Input: part model. Units: mm. Frame: model coordinates. A direction names the side the tool comes from. Round coordinates to 2 decimals unless told otherwise and drop trailing zeros. Loops run counter-clockwise (first coordinate to the right, second up) from the corner with the lowest first, then second, coordinate; pieces in that order, holes last.
1) Ray query, line 1 along Y through (x, z) = (0, 19); line 2 along X through (y, z) = (12.7, 40); line 3 along Y through (x, z) = (-2.5, 31). Return the intervals inside material, ascending.
2) Section B-B, the plane x = 3. Return loops of the section in (y, z), and give its area (3 significant figures).
3) Section D-D, the plane y = 17. Return loops of the section in (x, z), and give its area (3 significant figures).
4) Section A-A, the plane z = 41.5. Return loops of the section in (x, y).
5) Section C-C, the plane y = 21.5. Return loops of the section in (x, z).
6) Draft query along Y for faces 6 (the face through (0, 9.19, 36)), 7 (the face through (0, 27, 30)), 8 (the face through (0, 20.85, 36)). Return one class per face: pulls with the +Y half, pulls with the -Y half, needs draft (parallel to the pull), parting line crosses it, or undercut.
7) First-contact query: pin 1 (3 mm diameter, centred on y = 24.5, z = 33, fed in from -X); pin 2 (2 mm diameter, centred on x = 7, z = 7, fed in from -Y); pin 3 (3 mm diameter, centred on x = 4.5, y = 24.5, fed in from +Z); pin 4 (6 mm diameter, centred on x = 3, y = 19, fed in from -Z). Flat tips, straight axial feed; report the tip coordinate or a pass-through.
8) Access query for faces 1 (the face through (0, 14.85, 36)), 2 (the face through (0.657, 22.857, 12.325)), 3 (the face through (0, 9, 30)), 4 (the face through (-5, 24, 35)), 5 (the face through (0, 18, 30)). Directions: +Z, -Z, +X, -X, +Y, -Y. A direction counts if a zero-diameter tool reaches every point of the face in a straight line with its end or side. Return the directions, or none.
from build123d import *

# Parameters (mm, degrees)
SKETCH_1_R          = 10
EXTRUDE_1_DEPTH     = 30
SKETCH_2_W          = 10
SKETCH_2_H          = 17.320508075
EXTRUDE_3_DEPTH     = 15
CUT_EXTRUDE_1_DEPTH = 50.731328966
CUT_EXTRUDE_2_DEPTH = 50.731328966
CUT_EXTRUDE_3_DEPTH = 15
SKETCH_5_4_R        = 2.55
CUT_EXTRUDE_4_DEPTH = 50.731328966
SKETCH_9_R          = 5.05
CUT_EXTRUDE_5_DEPTH = 25


with BuildPart() as part:
    # Sketch 1 → Extrude 1 (new body)
    with BuildSketch(Plane.XY):
        with Locations((0, 17.850182559)):
            Circle(SKETCH_1_R)
    extrude(amount=EXTRUDE_1_DEPTH)

    # Sketch 2 → Extrude 3 (add)
    with BuildSketch(Plane.XY.offset(30)):
        with Locations((0, 17.85018256)):
            Rectangle(SKETCH_2_W, SKETCH_2_H)
    extrude(amount=EXTRUDE_3_DEPTH)

    # Sketch 5 → Cut-Extrude 1 (cut, through all)
    with BuildSketch(Plane(origin=(0, 26.510436597, 0), x_dir=(1, 0, 0), z_dir=(0, 1, 0))):
        with BuildLine():
            Line((5, -45), (5, -40))
            ThreePointArc((5, -40), (3.535533906, -43.535533906), (0, -45))
            Line((0, -45), (5, -45))
        make_face()
    extrude(amount=-CUT_EXTRUDE_1_DEPTH, mode=Mode.SUBTRACT)

    # Sketch 5_3 → Cut-Extrude 2 (cut, through all)
    with BuildSketch(Plane(origin=(0, 26.510436597, 0), x_dir=(1, 0, 0), z_dir=(0, 1, 0))):
        with BuildLine():
            ThreePointArc((0, -45), (-3.535533906, -43.535533906), (-5, -40))
            Line((-5, -40), (-5, -45))
            Line((-5, -45), (0, -45))
        make_face()
    extrude(amount=-CUT_EXTRUDE_2_DEPTH, mode=Mode.SUBTRACT)

    # Sketch 6 → Cut-Extrude 3 (cut)
    with BuildSketch(Plane(origin=(5, 0, 0), x_dir=(0, 0, -1), z_dir=(1, 0, 0))):
        Polygon((-40, 14.850182559), (-47.355991934, 14.850182559), (-47.355991934, 20.850182559), (-40, 20.850182559), (-30, 20.850182559), (-30, 14.850182559), align=None)
    extrude(amount=-CUT_EXTRUDE_3_DEPTH, mode=Mode.SUBTRACT)

    # Sketch 5_4 → Cut-Extrude 4 (cut, through all)
    with BuildSketch(Plane(origin=(0, 26.510436597, 0), x_dir=(1, 0, 0), z_dir=(0, 1, 0))):
        with Locations(Location((0, -40, 0), (0, 0, 270))):
            Circle(SKETCH_5_4_R)
    extrude(amount=-CUT_EXTRUDE_4_DEPTH, mode=Mode.SUBTRACT)

    # Sketch 9 → Cut-Extrude 5 (cut)
    with BuildSketch(Plane(origin=(0, 0, 0), x_dir=(-1, 0, 0), z_dir=(0, 0, -1))):
        with Locations((0, 17.850182559)):
            Circle(SKETCH_9_R)
    extrude(amount=-CUT_EXTRUDE_5_DEPTH, mode=Mode.SUBTRACT)


solid = part.part
Final values:
1. line 1: y = 7.85 to 12.8, 22.9 to 27.85
1. line 2: x = -5 to -2.55, 2.55 to 5
1. line 3: y = 9.19 to 14.85, 20.85 to 26.51
2. outline: (8.31, 0) - (13.79, 0) - (13.79, 25) - (21.91, 25) - (21.91, 0) - (27.39, 0) - (27.39, 30) - (26.51, 30) - (26.51, 44) - (20.85, 44) - (20.85, 30) - (14.85, 30) - (14.85, 44) - (9.19, 44) - (9.19, 30) - (8.31, 30) - close
2. area: 528 mm2
3. outline: (-9.96, 0) - (-4.98, 0) - (-4.98, 25) - (4.98, 25) - (4.98, 0) - (9.96, 0) - (9.96, 30) - (-9.96, 30) - close
3. area: 349 mm2
4. outline: (-4.77, 9.19) - (-2.06, 9.19) - (-2.06, 14.85) - (-4.77, 14.85) - close; (-4.77, 20.85) - (-2.06, 20.85) - (-2.06, 26.51) - (-4.77, 26.51) - close; (2.06, 9.19) - (4.77, 9.19) - (4.77, 14.85) - (2.06, 14.85) - close; (2.06, 20.85) - (4.77, 20.85) - (4.77, 26.51) - (2.06, 26.51) - close
5. outline: (-9.31, 0) - (-3.49, 0) - (-3.49, 25) - (3.49, 25) - (3.49, 0) - (9.31, 0) - (9.31, 30) - (5, 30) - (5, 40) arc R5 ccw to (-5, 40) - (-5, 30) - (-9.31, 30) - close; hole circle Ø5.1 at (0, 40)
6. face 6: pulls with the -Y half
6. face 7: needs draft
6. face 8: undercut
7. pin 1: stops at x = -5
7. pin 2: stops at y = 9.85
7. pin 3: stops at z = 44
7. pin 4: stops at z = 0
8. face 1: +Z, +X, -X
8. face 2: -Z
8. face 3: +Z, +X, -X, -Y
8. face 4: +Z, -X, +Y, -Y
8. face 5: +Z
